```python
from build123d import *

# Parameters (mm, degrees)
F0_R     = 6.984327
F0_R_2   = 3.175
F0_R_3   = 3.727636
F1_DEPTH = 101.6


with BuildPart() as f1:
    # F0 (on Front) → F1 (new body)
    with BuildSketch(Plane.XZ):
        with BuildLine():
            ThreePointArc((15.826897, -1.234892), (15.86297, -0.617914), (15.875, 0))
            ThreePointArc((15.875, 0), (15.843841, 0.994139), (15.750488, 1.984375))
            ThreePointArc((15.750488, 1.984375), (0, 15.875), (-15.750488, 1.984375))
            ThreePointArc((-15.750488, 1.984375), (-15.873744, 0.199705), (-15.795426, -1.5875))
            ThreePointArc((-15.795426, -1.5875), (0.177005, -15.874013), (15.826897, -1.234892))
        make_face()
        Circle(F0_R, mode=Mode.SUBTRACT)
        with BuildLine():
            ThreePointArc((-15.750488, 1.984375), (0, 15.875), (15.750488, 1.984375))
            Line((15.750488, 1.984375), (9.450293, 51.990625))
            ThreePointArc((9.450293, 51.990625), (9.506305, 51.396483), (9.525, 50.8))
            ThreePointArc((9.525, 50.8), (-0.596483, 41.293695), (-9.450293, 51.990625))
            Line((-9.450293, 51.990625), (-15.750488, 1.984375))
        make_face()
        with Locations((-3.175, 36.5252)):
            Circle(F0_R_2, mode=Mode.SUBTRACT)
        with BuildLine():
            Line((11.464128, -57.15), (15.826897, -1.234892))
            ThreePointArc((15.826897, -1.234892), (0.177005, -15.874013), (-15.795426, -1.5875))
            Line((-15.795426, -1.5875), (-9.477255, -64.4525))
            ThreePointArc((-9.477255, -64.4525), (-0.476848, -53.986944), (9.525, -63.5))
            ThreePointArc((9.525, -63.5), (6.735192, -70.235192), (0, -73.025))
            Line((0, -73.025), (44.45, -73.025))
            ThreePointArc((44.45, -73.025), (36.5125, -65.0875), (44.45, -57.15))
            Line((44.45, -57.15), (11.464128, -57.15))
        make_face()
        with BuildLine():
            ThreePointArc((9.525, 50.8), (9.506305, 51.396483), (9.450293, 51.990625))
            ThreePointArc((9.450293, 51.990625), (0, 60.325), (-9.450293, 51.990625))
            ThreePointArc((-9.450293, 51.990625), (-0.596483, 41.293695), (9.525, 50.8))
        make_face()
        with Locations((0, 50.8)):
            Circle(F0_R_2, mode=Mode.SUBTRACT)
        with BuildLine():
            ThreePointArc((9.525, -63.5), (-0.476848, -53.986944), (-9.477255, -64.4525))
            ThreePointArc((-9.477255, -64.4525), (-6.389564, -70.563929), (0, -73.025))
            ThreePointArc((0, -73.025), (6.735192, -70.235192), (9.525, -63.5))
        make_face()
        with Locations((0, -63.5)):
            Circle(F0_R_3, mode=Mode.SUBTRACT)
        with BuildLine():
            ThreePointArc((52.3875, -65.0875), (50.06266, -59.47484), (44.45, -57.15))
            ThreePointArc((44.45, -57.15), (36.5125, -65.0875), (44.45, -73.025))
            ThreePointArc((44.45, -73.025), (50.06266, -70.70016), (52.3875, -65.0875))
        make_face()
        with Locations((44.45, -65.0875)):
            Circle(F0_R_3, mode=Mode.SUBTRACT)
    extrude(amount=F1_DEPTH)


solid = f1.part
```
Geometry: final body of the model. Coordinates: model frame, mm. A direction names the side the tool comes from. Give positions to 0.01 mm unless a question says otherwise; leave off trailing zeros. Write each loop counter-clockwise with the first axis right and the second up, starting at its lowest first coordinate (ties: lowest second). Pieces come first, ordered by that corner, then holes.
1. Section query C-C, the plane z = 26. Return loops of the section in (x, y).
2. Reachability of faces 1 (the flat face through (13.615, -50.089, -29.584)), 2 (the flat face through (12.644, -50.089, 26.637)) from +Z, -Z, +X, -X, +Y, -Y: full face, straight path, thin tool, end or side. Return the list, or none.
3. Section query A-A, the plane y = -28.5. Count the separate pieces of the cut face and the enclosed holes in it, then the cut area to 3 significant figures.
4. Line query: probe 1 along Z at (x, y) = (-1, -83); probe 2 along Z at (x, y) = (44, -41) (3 decimals); probe 3 along Z at (x, y) = (42.5, -59) (3 decimals). Output: solid intervals per line, ascending.
5. Section query B-B, the plane x = 31.5. Return loops of the section in (y, z) (3 decimals).
6. Draft query along Z for faces 3 (the cylindrical face through (0.193, -50.089, 60.323)), 4 (the cylindrical face through (-6.46, -50.09, -70.5)), 5 (the cylindrical face through (-0.81, -50.09, -67.14)). Return one class per face: released by +Z, released by -Z, zero draft, split by the parting line, or undercut.
7. Pin query (flat end, axial travel): P1, Ø1, axis at x = 17.5, z = -56, coming from the +Y side. Return the tip coordinate at first contact, or that it passes through.
Computed:
1. outline: (-12.72, -101.6) - (12.72, -101.6) - (12.72, 0) - (-12.72, 0) - close
2. face 1: +X, +Y, -Y
2. face 2: +Z, +X, +Y, -Y
3. separate pieces: 1
3. enclosed holes: 5
3. area: 3,610 mm2
4. probe 1: z = -72.97 to -67.09, -59.91 to -6.91, 6.91 to 34.21, 38.84 to 47.79, 53.81 to 60.27
4. probe 2: z = -73.025 to -68.788, -61.387 to -57.15
4. probe 3: z = -73.025 to -68.264, -61.911 to -57.15
5. outline: (-101.6, -73.025) - (0, -73.025) - (0, -57.15) - (-101.6, -57.15) - close
6. face 3: released by +Z
6. face 4: released by -Z
6. face 5: undercut
7. P1: passes through
